```python
from build123d import *

# Parameters (mm, degrees)
F1_DEPTH = 44.958


with BuildPart() as f1:
    # F0 (on Right) → F1 (new body)
    with BuildSketch(Plane.YZ):
        with BuildLine():
            Line((19.538479, -23.200311), (13.070115, -23.200311))
            ThreePointArc((13.070115, -23.200311), (0, -36.270426), (-13.070115, -23.200311))
            Line((-13.070115, -23.200311), (-19.538479, -23.200311))
            ThreePointArc((-19.538479, -23.200311), (0, -42.73879), (19.538479, -23.200311))
        make_face()
        with BuildLine():
            ThreePointArc((-13.070115, -23.200311), (0, -10.130196), (13.070115, -23.200311))
            Line((13.070115, -23.200311), (19.538479, -23.200311))
            ThreePointArc((19.538479, -23.200311), (0, -3.661832), (-19.538479, -23.200311))
            Line((-19.538479, -23.200311), (-13.070115, -23.200311))
        make_face()
        with BuildLine():
            ThreePointArc((-19.538479, -23.200311), (0, -3.661832), (19.538479, -23.200311))
            Line((19.538479, -23.200311), (19.538479, 23.200311))
            Line((19.538479, 23.200311), (-19.538479, 23.200311))
            Line((-19.538479, 23.200311), (-19.538479, -23.200311))
        make_face()
    extrude(amount=F1_DEPTH)


solid = f1.part
```
Work out the finished part from the listing and answer in its coordinate system (mm). Give positions to 0.01 mm unless a question says otherwise; leave off trailing zeros. Write each loop counter-clockwise with the first axis right and the second up, starting at its lowest first coordinate (ties: lowest second). Pieces come first, ordered by that corner, then holes.
(1) The mould has two halves that part along Y. Classify faces 1 (the flat face through (22, 19.538, 0)), 2 (the cylindrical face through (22.164, 13.057, -22.626)), 3 (the flat face through (0, 0, -2)): pulls with the +Y half, pulls with the -Y half, needs draft (parallel to the pull), parting line crosses it, or undercut.
Final values:
face 1: pulls with the +Y half
face 2: undercut
face 3: needs draft
(2) The part is cut by section A-A on y = 0. Write down the section's boundary in (x, z).
Final values:
outline: (0, -42.74) - (44.96, -42.74) - (44.96, -36.27) - (0, -36.27) - close; (0, -10.13) - (44.96, -10.13) - (44.96, 23.2) - (0, 23.2) - close
(3) Flat-ended cylindrical pins translate along their axes: pin 1 Ø6 at (x, y) = (36.5, -6.5) entering from -Z; pin 2 Ø8 at (x, z) = (11, -32.5) entering from +Y; pin 3 Ø3 at (x, z) = (22, -27.5) entering from +Y. Find the tip coordinate at first contact, or state that the pin passes through.
Final values:
pin 1: stops at z = -42.42
pin 2: stops at y = 18.81
pin 3: stops at y = 19.34
(4) The part is cut by section C-C on x = 36.5. Write down the section's boundary in (y, z), plus the area to 3 significant figures.
Final values:
outline: (-19.54, -23.2) arc R19.54 ccw to (19.54, -23.2) - (19.54, 23.2) - (-19.54, 23.2) - close; hole circle Ø26.14 at (0, -23.2)
area: 1,880 mm2
(5) The part is cut by section B-B on z = -35. Write down the section's boundary in (x, y).
Final values:
outline: (0, -15.57) - (44.96, -15.57) - (44.96, -5.62) - (0, -5.62) - close; (0, 5.62) - (44.96, 5.62) - (44.96, 15.57) - (0, 15.57) - close
(6) The part is cut by section D-D on y = 14. Write down the section's boundary in (x, z).
Final values:
outline: (0, -36.83) - (44.96, -36.83) - (44.96, 23.2) - (0, 23.2) - close
(7) Straight lines are drawn through the part: line 1 (Z direction, x = 16, y = 0); line 2 (Y direction, x = 32, z = -23); line 3 (Y direction, x = 16, z = -34). For each, find the intervals that lie inside material, in ascending order.
Final values:
line 1: z = -42.74 to -36.27, -10.13 to 23.2
line 2: y = -19.54 to -13.07, 13.07 to 19.54
line 3: y = -16.28 to -7.36, 7.36 to 16.28
